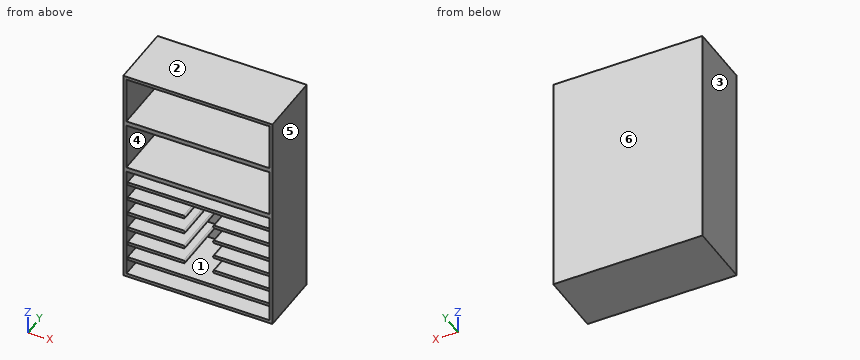
from build123d import *

# Parameters (mm, degrees)
F0_W     = 609.6
F0_H     = 914.4
F1_DEPTH = 263.525
F2_T     = -12.7
F3_W     = 584.2
F3_H     = 19.05
F4_DEPTH = 250.825
F6_DEPTH = 241.3
F7_DEPTH = 241.3


# Not quite as in the source:
# - a feature names something its author has since deleted; it is built from what else it names


with BuildPart() as f1:
    # F0 (on Front) → F1 (new body)
    with BuildSketch(Plane.XZ):
        Rectangle(F0_W, F0_H)
    extrude(amount=F1_DEPTH)

    # F2
    f2_openings = [f1.faces().sort_by_distance(p)[0] for p in [
        (0, -263.525, 0),
    ]]
    offset(amount=F2_T, openings=f2_openings)

    # F3 (on face) → F4 (join)
    with BuildSketch(Plane.XZ.offset(12.7)):
        with Locations((0, 32.385)):
            Rectangle(F3_W, F3_H)
        with Locations((0, 243.205)):
            Rectangle(F3_W, F3_H)
    extrude(amount=F4_DEPTH)

    # F5 (on face) → F6 (join)
    with BuildSketch(Plane.XZ.offset(12.7)):
        Polygon((-63.5, -33.02), (-292.1, -33.02), (-292.1, -45.72), (-63.5, -45.72), (63.5, -45.72), (292.1, -45.72), (292.1, -33.02), (63.5, -33.02), align=None)
    extrude(amount=F6_DEPTH)

    # F5 (on face) → F7 (join)
    with BuildSketch(Plane.XZ.offset(12.7)):
        with BuildLine():
            Line((292.1, -182.88), (292.1, -170.18))
            Line((292.1, -170.18), (63.5, -170.18))
            ThreePointArc((63.5, -170.18), (57.15, -176.53), (63.5, -182.88))
            Line((63.5, -182.88), (292.1, -182.88))
        make_face()
        with BuildLine():
            Line((292.1, -114.3), (292.1, -101.6))
            Line((292.1, -101.6), (63.5, -101.6))
            ThreePointArc((63.5, -101.6), (57.15, -107.95), (63.5, -114.3))
            Line((63.5, -114.3), (292.1, -114.3))
        make_face()
        Polygon((-63.5, -33.02), (-292.1, -33.02), (-292.1, -45.72), (-63.5, -45.72), (63.5, -45.72), (292.1, -45.72), (292.1, -33.02), (63.5, -33.02), align=None)
        with BuildLine():
            Line((-63.5, -170.18), (-292.1, -170.18))
            Line((-292.1, -170.18), (-292.1, -182.88))
            Line((-292.1, -182.88), (-63.5, -182.88))
            ThreePointArc((-63.5, -182.88), (-57.15, -176.53), (-63.5, -170.18))
        make_face()
        with BuildLine():
            Line((-63.5, -101.6), (-292.1, -101.6))
            Line((-292.1, -101.6), (-292.1, -114.3))
            Line((-292.1, -114.3), (-63.5, -114.3))
            ThreePointArc((-63.5, -114.3), (-57.15, -107.95), (-63.5, -101.6))
        make_face()
        with BuildLine():
            Line((-63.5, -238.76), (-292.1, -238.76))
            Line((-292.1, -238.76), (-292.1, -251.46))
            Line((-292.1, -251.46), (-63.5, -251.46))
            ThreePointArc((-63.5, -251.46), (-57.15, -245.11), (-63.5, -238.76))
        make_face()
        with BuildLine():
            Line((292.1, -251.46), (292.1, -238.76))
            Line((292.1, -238.76), (63.5, -238.76))
            ThreePointArc((63.5, -238.76), (57.15, -245.11), (63.5, -251.46))
            Line((63.5, -251.46), (292.1, -251.46))
        make_face()
        with BuildLine():
            Line((292.1, -320.04), (292.1, -307.34))
            Line((292.1, -307.34), (63.5, -307.34))
            ThreePointArc((63.5, -307.34), (57.15, -313.69), (63.5, -320.04))
            Line((63.5, -320.04), (292.1, -320.04))
        make_face()
        with BuildLine():
            Line((-63.5, -307.34), (-292.1, -307.34))
            Line((-292.1, -307.34), (-292.1, -320.04))
            Line((-292.1, -320.04), (-63.5, -320.04))
            ThreePointArc((-63.5, -320.04), (-57.15, -313.69), (-63.5, -307.34))
        make_face()
        Polygon((-63.5, -375.92), (-292.1, -375.92), (-292.1, -388.62), (-63.5, -388.62), (63.5, -388.62), (292.1, -388.62), (292.1, -375.92), (63.5, -375.92), align=None)
    extrude(amount=F7_DEPTH)


solid = f1.part
Part model, mm, in its own coordinate system. Face numbers are marked on the shaded views. A direction names the side the tool comes from. Coordinates: 2 decimals unless noted, no trailing zeros. Loops run counter-clockwise (first coordinate to the right, second up) from the corner with the lowest first, then second, coordinate; pieces in that order, holes last. Notation, with made-up numbers: M 56,27.25 L 87,27.25 A19 ccw 87,52.25 Z; hole C 55,76 d5. An arc over 180 degrees is marked long. Use a Markdown table: item, result. Add a question column.
Q1. Which spindle directions (+Z, -Z, +X, -X, +Y, -Y) get a long thin tool onto all of the face, cutting with end or side? Do the marked faces 1 and 2. Say none if no direction does.
Q2. Cut at B-B (y = -88). Give the number of separate pieces and of enclosed holes in the cut face, and give its area (3 significant figures).
Q3. Mould opens along X. For the marked faces 3, 4, 5 and 6 say: +X half, -X half, draft (parallel to the pull), parting line (faces both ways), or undercut.
Q4. Probe L1, parallel to Z at x = -20.5, y = -15; L2, parallel to X at y = -33, z = 398; L3, parallel to X at y = -146.5, z = -313.5. List the from-to ranges inside material, lowest first.
Q5. Cut at A-A (z = -334.5). Write the cut outline in (x, y) (3 decimals), and give its area (3 significant figures).
Q6. Pin check, flat tip, straight feed: P1, Ø10, axis at x = 159, z = -311.5, coming from the -Y side. Stop position of the tip, or through.
Worked out:
| question | item | result |
|---|---|---|
| 1 | face 1 | -Y |
| 1 | face 2 | +Z, +X, -X, +Y, -Y |
| 2 | separate pieces | 1 |
| 2 | enclosed holes | 5 |
| 2 | area | 98,900 mm2 |
| 3 | face 3 | -X half |
| 3 | face 4 | undercut |
| 3 | face 5 | +X half |
| 3 | face 6 | draft |
| 4 | L1 | z = -457.2 to -444.5, -388.62 to -375.92, -45.72 to -33.02, 22.86 to 41.91, 233.68 to 252.73, 444.5 to 457.2 |
| 4 | L2 | x = -304.8 to -292.1, 292.1 to 304.8 |
| 4 | L3 | x = -304.8 to -57.15, 57.15 to 304.8 |
| 5 | outline | M -304.8,-263.525 L -292.1,-263.525 L -292.1,-12.7 L 292.1,-12.7 L 292.1,-263.525 L 304.8,-263.525 L 304.8,0 L -304.8,0 Z |
| 5 | area | 14,100 mm2 |
| 6 | P1 | stops at y = -254 |
